Geometry: final body of the model. Coordinates: model frame, mm. Round coordinates to 2 decimals unless told otherwise and drop trailing zeros. Loops run counter-clockwise (first coordinate to the right, second up) from the corner with the lowest first, then second, coordinate; pieces in that order, holes last. Notation, with made-up numbers: (9.25, 68) - (17.25, 68) arc R21 cw to (17.25, 82) - close; hole circle Ø5 at (-29.5, -26.75). An arc over 180 degrees is marked (long way). Answer as CSV lines item,"result".
Autodesk Inventor part; units mm, degrees
ref_plane "YZ Plane" through (0, 0, 0) normal (1, 0, 0) x (0, 1, 0)
ref_plane "XZ Plane" through (0, 0, 0) normal (0, 1, 0) x (-1, 0, 0)
ref_plane "XY Plane" through (0, 0, 0) normal (0, 0, 1) x (1, 0, 0)
ref_plane "Plano de trabalho1" through (0, 142, 0) normal (0, 0, 1) x (0, -1, 0)
sketch "Esboço1" plane through (0, 142, 0) normal (0, 0, 1) x (0, -1, 0)
  arc A0 (124, -4) -> (125, -5) centre (125, -4) ccw
  line L0 (142, -5) -> (125, -5)
  line L1 (142, -5) -> (142, -8)
  line L2 (142, -8) -> (144, -8)
  arc A1 (144, -8) -> (150, -2) centre (144, -2) ccw
  line L3 (150, -2) -> (150, 0)
  line L4 (150, 0) -> (147, 0)
  line L5 (147, 0) -> (147, 17)
  arc A2 (147, 17) -> (146, 18) centre (146, 17) ccw
  line L6 (135, 18) -> (146, 18)
  arc A3 (135, 18) -> (134, 17) centre (135, 17) ccw
  line L7 (134, 9) -> (134, 17)
  arc A4 (133, 8) -> (134, 9) centre (133, 9) ccw
  line L8 (133, 8) -> (124, 8)
  line L9 (124, -4) -> (124, 8)
  circle A5 centre (141, 13) radius 2
  circle A6 centre (129, 2) radius 2
  arc A7 (-4, 18) -> (-5, 17) centre (-4, 17) ccw
  line L10 (-5, 0) -> (-5, 17)
  line L11 (-5, 0) -> (-8, 0)
  line L12 (-8, 0) -> (-8, -2)
  arc A8 (-8, -2) -> (-2, -8) centre (-2, -2) ccw
  line L13 (-2, -8) -> (0, -8)
  line L14 (0, -8) -> (0, -5)
  line L15 (0, -5) -> (17, -5)
  arc A9 (17, -5) -> (18, -4) centre (17, -4) ccw
  line L16 (18, 7) -> (18, -4)
  arc A10 (18, 7) -> (17, 8) centre (17, 7) ccw
  line L17 (9, 8) -> (17, 8)
  arc A11 (8, 9) -> (9, 8) centre (9, 9) ccw
  line L18 (8, 9) -> (8, 18)
  line L19 (-4, 18) -> (8, 18)
  circle A12 centre (13, 1) radius 2
  circle A13 centre (2, 13) radius 2
  circle A14 centre (141, 110) radius 2
  circle A15 centre (129, 121) radius 2
  arc A16 (146, 105) -> (147, 106) centre (146, 106) ccw
  line L20 (147, 123) -> (147, 106)
  line L21 (150, 123) -> (147, 123)
  line L22 (150, 125) -> (150, 123)
  arc A17 (150, 125) -> (144, 131) centre (144, 125) ccw
  line L23 (144, 131) -> (124, 131)
  line L24 (124, 116) -> (124, 131)
  arc A18 (124, 116) -> (125, 115) centre (125, 116) ccw
  line L25 (133, 115) -> (125, 115)
  arc A19 (134, 114) -> (133, 115) centre (133, 114) ccw
  line L26 (134, 114) -> (134, 106)
  arc A20 (134, 106) -> (135, 105) centre (135, 106) ccw
  line L27 (146, 105) -> (135, 105)
  arc A21 (17, 115) -> (18, 116) centre (17, 116) ccw
  line L28 (18, 131) -> (18, 116)
  line L29 (-2, 131) -> (18, 131)
  arc A22 (-2, 131) -> (-8, 125) centre (-2, 125) ccw
  line L30 (-8, 125) -> (-8, 123)
  line L31 (-8, 123) -> (-5, 123)
  line L32 (-5, 123) -> (-5, 106)
  arc A23 (-5, 106) -> (-4, 105) centre (-4, 106) ccw
  line L33 (7, 105) -> (-4, 105)
  arc A24 (7, 105) -> (8, 106) centre (7, 106) ccw
  line L34 (8, 114) -> (8, 106)
  arc A25 (9, 115) -> (8, 114) centre (9, 114) ccw
  line L35 (9, 115) -> (17, 115)
  circle A26 centre (1, 110) radius 2
  circle A27 centre (13, 121) radius 2
  line L36 (18, 131) -> (124.2929, 131)
  line L37 (150, 123) -> (150, 0)
  line L38 (0, -8) -> (142, -8)
  line L39 (-8, 0) -> (-8, 123)
  point P0 (142, 0)
extrude "Extrusão1" add sketch "Esboço1" along normal blind 4
sketch "Esboço2" plane through (0, 142, 4) normal (0, 0, 1) x (1, 0, 0)
  circle A0 centre (61.5, -17.9015) radius 5
  circle A1 centre (61.5, -124.1015) radius 5
  circle A2 centre (61.7717, -71.0022) radius 5.8
  circle A3 centre (61.5, -45.0015) radius 2.1
  circle A4 centre (61.5, -97.0015) radius 2.1
  circle A5 centre (61.5, -17.9015) radius 5.05
  circle A6 centre (61.5, -45.0015) radius 2.1
  circle A7 centre (61.5, -97.0015) radius 2.1
  circle A8 centre (61.7717, -71.0022) radius 1.5
  circle A9 centre (61.5, -124.1015) radius 5
  point P0 (0, -142)
  dimension "d2" = 10.1
  dimension "d3" = 4.2
  dimension "d4" = 3
  dimension "d19" = 10
extrude "Extrusão2" cut sketch "Esboço2" against normal blind 4 contours A0 | A1 | A3 | A4 | A8
sketch "Esboço3" plane through (0, 142, 4) normal (0, 0, 1) x (1, 0, 0)
  circle A0 centre (61.5, -124.1015) radius 5
  circle A1 centre (61.5, -124.1015) radius 16
  circle A2 centre (61.5, -17.9015) radius 5
  circle A3 centre (61.5, -17.9015) radius 16
  line L0 (45.5, -17.9015) -> (77.5, -17.9015)
  line L1 (45.5, -124.1015) -> (77.5, -124.1015)
  circle A4 centre (77.5, -124.1015) radius 2.1
  circle A5 centre (45.5, -124.1015) radius 2.1
  circle A6 centre (77.5, -17.9015) radius 2.1
  circle A7 centre (45.5, -17.9015) radius 2.1
  point P0 (0, -142)
  dimension "d7" = 32
  dimension "d8" = 32
  dimension "d9" = 4.2
  dimension "d10" = 4.2
  dimension "d11" = 4.2
  dimension "d12" = 4.2
extrude "Extrusão3" cut sketch "Esboço3" against normal blind 4 contours A4 A1 L1 | L1 A1 A4 | A5 A1 L1 | L1 A1 A5 | A1 A4 | A1 A5 | A6 A3 L0 | L0 A3 A6 | A7 A3 L0 | L0 A3 A7 | A3 A6 | A3 A7
sketch "Esboço4" plane through (0, 142, 0) normal (0, 0, -1) x (-1, 0, 0)
  circle A0 centre (-90.5, -93.0015) radius 2.1
  circle A1 centre (-90.5, -49.0015) radius 2.1
  point P0 (0, -142)
  dimension "d15" = 4.2
  dimension "d16" = 4.2
extrude "Extrusão4" cut sketch "Esboço4" against normal blind 4
sketch "Esboço5" plane through (0, 142, 4) normal (0, 0, 1) x (1, 0, 0)
  circle A0 centre (61.5, -124.1015) radius 5
  circle A1 centre (61.5, -124.1015) radius 5.05
  circle A2 centre (61.5, -17.9015) radius 5
  circle A3 centre (61.5, -17.9015) radius 5.05
  point P0 (0, -142)
  dimension "d20" = 10.1
  dimension "d21" = 10.1
extrude "Extrusão5" cut sketch "Esboço5" against normal blind 10
properties part number "fechamentocima"
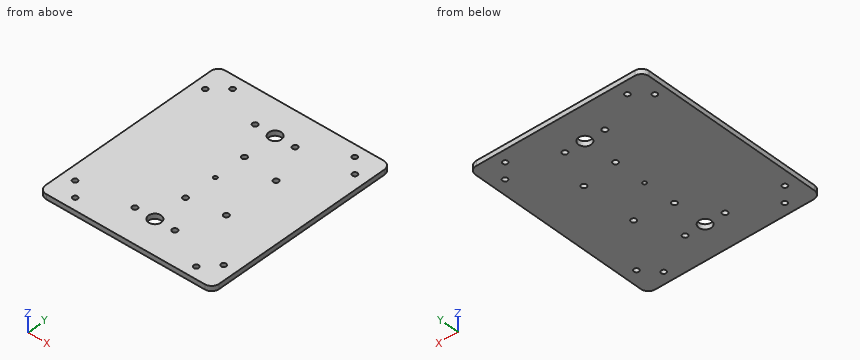
(1) Material intervals for line 1 along Y through (x, z) = (61.5, 2.15); line 2 along Y through (x, z) = (77.5, 1); line 3 along Y through (x, z) = (44, 0.3), sorted ascending.
Findings below:
line 1,"-8 to 12.85, 22.95 to 42.9, 47.1 to 69.52, 72.47 to 94.9, 99.1 to 119.05, 129.15 to 150"
line 2,"-8 to 15.8, 20 to 122, 126.2 to 150"
line 3,"-8 to 16.43, 19.37 to 122.63, 125.57 to 150"
(2) Section B-B (y = 1). Output: boundary loops of the cut face in (x, z).
Findings below:
outline,"(-8, 0) - (11, 0) - (11, 4) - (-8, 4) - close; (15, 0) - (108, 0) - (108, 4) - (15, 4) - close; (112, 0) - (131, 0) - (131, 4) - (112, 4) - close"
(3) Section A-A (x = 90.5). Output: boundary loops of the cut face in (y, z), and give its area (3 significant figures).
Findings below:
outline,"(-8, 0) - (46.9, 0) - (46.9, 4) - (-8, 4) - close; (51.1, 0) - (90.9, 0) - (90.9, 4) - (51.1, 4) - close; (95.1, 0) - (150, 0) - (150, 4) - (95.1, 4) - close"
area,"598 mm2"
(4) Section C-C (z = 2.7). Give the number of separate pieces and of enclosed holes in the cut face, and give its area (3 significant figures).
Findings below:
separate pieces,"1"
enclosed holes,"19"
area,"21,600 mm2"
(5) Pin query (flat end, axial travel): P1, Ø4, axis at x = 45.5, y = 17.9, coming from the +Z side. Return the tip coordinate at first contact, or that it passes through.
Findings below:
P1,"through"
